Geometry check sheet. Reference: the model listing, model coordinates, mm. A direction names the side the tool comes from. Round coordinates to 2 decimals unless told otherwise and drop trailing zeros. One line per question, with ' | ' between items.
```python
from build123d import *

# Parameters (mm, degrees)
PAD033_DEPTH    = 3
PAD033_TAPER    = 14
SKETCH057_R     = 2
PAD034_DEPTH    = 4
POCKET008_DEPTH = 4.6
POCKET008_TAPER = 15
POCKET009_DEPTH = 2
SKETCH056_W     = 11
SKETCH056_H     = 3
POCKET010_DEPTH = 5


with BuildPart() as part:
    # Sketch055 → Pad033 (new body)
    with BuildSketch(Plane.XY.offset(-4)):
        with BuildLine():
            ThreePointArc((-17.734351, 11.23491), (-16.243686, 13.811706), (-14.965, 16.5))
            Line((-14.965, 16.5), (14.965, 16.5))
            ThreePointArc((14.965, 16.5), (16.243686, 13.811706), (17.734351, 11.23491))
            ThreePointArc((12.98, -16.5), (20.691765, -3.547007), (17.734351, 11.23491))
            Line((-12.98, -16.5), (12.98, -16.5))
            ThreePointArc((-17.734351, 11.23491), (-20.691765, -3.547007), (-12.98, -16.5))
        make_face()
    extrude(amount=-PAD033_DEPTH, taper=PAD033_TAPER)

    # Sketch057 → Pad034 (join)
    with BuildSketch(Plane.XY):
        with BuildLine():
            ThreePointArc((13.586881, 20.251823), (12.228055, 23.328699), (10.184105, 26))
            Line((-10.184105, 26), (10.184105, 26))
            ThreePointArc((-10.184105, 26), (-12.228055, 23.328699), (-13.586881, 20.251823))
            ThreePointArc((-17.728491, 11.256137), (-15.355357, 15.614788), (-13.586881, 20.251823))
            ThreePointArc((-17.728491, 11.256137), (-20.699674, -3.538854), (-12.982142, -16.506483))
            ThreePointArc((-6.502297, -26.893782), (-8.833051, -21.132971), (-12.982142, -16.506483))
            ThreePointArc((-6.502297, -26.893782), (0, -32.15), (6.502297, -26.893782))
            ThreePointArc((12.982142, -16.506483), (8.833051, -21.132971), (6.502297, -26.893782))
            ThreePointArc((12.982142, -16.506483), (20.699674, -3.538854), (17.728491, 11.256137))
            ThreePointArc((13.586881, 20.251823), (15.355357, 15.614788), (17.728491, 11.256137))
        make_face()
        with Locations((0, -25.5)):
            Circle(SKETCH057_R, mode=Mode.SUBTRACT)
        with Locations((-8, 21.5)):
            Circle(SKETCH057_R, mode=Mode.SUBTRACT)
        with Locations((8, 21.5)):
            Circle(SKETCH057_R, mode=Mode.SUBTRACT)
    extrude(amount=-PAD034_DEPTH)

    # Sketch058 → Pocket008 (cut)
    with BuildSketch(Plane.XY):
        with BuildLine():
            Line((-14.85, 11.05), (-14.85, -10.95))
            ThreePointArc((-14.85, -10.95), (-13.649138, -13.849138), (-10.75, -15.05))
            Line((-10.75, -15.05), (10.85, -15.05))
            ThreePointArc((10.85, -15.05), (13.678427, -13.878427), (14.85, -11.05))
            Line((14.85, -11.05), (14.85, 11.05))
            ThreePointArc((14.85, 11.05), (13.678427, 13.878427), (10.85, 15.05))
            Line((10.85, 15.05), (-10.85, 15.05))
            ThreePointArc((-10.85, 15.05), (-13.678427, 13.878427), (-14.85, 11.05))
        make_face()
    extrude(amount=-POCKET008_DEPTH, taper=POCKET008_TAPER, mode=Mode.SUBTRACT)

    # Sketch025 (on Face20 of Pocket008) → Pocket009 (cut)
    with BuildSketch(Plane(origin=(0, -3.3492, -4), x_dir=(1, 0, 0), z_dir=(0, 0, 1))):
        Polygon((12, 24.9), (10, 28.364102), (6, 28.364102), (4, 24.9), (6, 21.435898), (10, 21.435898), align=None)
        Polygon((-4, 24.9), (-6, 28.364102), (-10, 28.364102), (-12, 24.9), (-10, 21.435898), (-6, 21.435898), align=None)
        Polygon((4, -22.1), (2, -18.635898), (-2, -18.635898), (-4, -22.1), (-2, -25.564102), (2, -25.564102), align=None)
    extrude(amount=POCKET009_DEPTH, mode=Mode.SUBTRACT)

    # Sketch056 → Pocket010 (cut)
    with BuildSketch(Plane.XY.offset(-4)):
        with Locations((0, 9.5)):
            Rectangle(SKETCH056_W, SKETCH056_H)
    extrude(amount=-POCKET010_DEPTH, mode=Mode.SUBTRACT)


with BuildPart() as part_1:
    # Body016 placement: moved
    add(part.part.moved(Location((0, 0, -10))))


solid = part_1.part
```
(1) Draft check along X on faces 1 (the cylindrical face through (-8.787, -21.207, -11.972)), 2 (the flat face through (11.014, 23.259, -13.014)), 3 (the flat face through (0, 26, -12)), 4 (the flat face through (-4.986, 23.259, -13.014)). Enter one of: +X half, -X half, draft (parallel to the pull), parting line (faces both ways), or undercut.
Resolved:
face 1: -X half | face 2: undercut | face 3: draft | face 4: undercut
(2) Go/stop test with flat-tipped pins: pin 1 (2.5 mm diameter, centred on x = -1.5, z = -16.5, fed in from +Y); pin 2 (4 mm diameter, centred on x = 12.5, z = -14, fed in from -Y); pin 3 (1.9 mm diameter, centred on y = 9, z = -15.5, fed in from -X). Record where each tip stops, or that it passes through.
Resolved:
pin 1: stops at y = 16.19 | pin 2: stops at y = -18.87 | pin 3: stops at x = -19.06
(3) Material ranges on line 1 (Z direction, x = 5, y = -11.5); line 2 (Z direction, x = 8.5, y = 17); line 3 (Y direction, x = -8, z = -11.6), recorded low to high.
Resolved:
line 1: z = -17 to -14.6 | line 2: z = -14 to -10 | line 3: y = -22.62 to -14.62, 14.62 to 19.5, 23.5 to 26
(4) Access from +Z, -Z, +X, -X, +Y, -Y to the whole of each face (thin tool, end or side, straight path). Record for faces 5 (the flat face through (0, 20, -14)), 6 (the flat face through (5.014, 23.307, -13.014)), 7 (the flat face through (0, 8, -16)).
Resolved:
face 5: -Z, +X, -X, +Y | face 6: -Z | face 7: +Z, -Z
(5) Sectioned sample at A-A on x = 0. Count the separate pieces of the cut face and the enclosed holes in it, then the cut area to 3 significant figures.
Resolved:
separate pieces: 3 | enclosed holes: 0 | area: 168 mm2
